from build123d import *

# Parameters (mm, degrees)
F1_W     = 106
F1_H     = 44
F1_W_2   = 100
F1_H_2   = 38
F2_DEPTH = 40
F3_W     = 106
F3_H     = 44
F3_W_2   = 100
F3_H_2   = 38
F4_DEPTH = 3


with BuildPart() as f2:
    # F1 (on Top) → F2 (new body)
    with BuildSketch(Plane.XY):
        Rectangle(F1_W, F1_H)
        Rectangle(F1_W_2, F1_H_2, mode=Mode.SUBTRACT)
    extrude(amount=-F2_DEPTH)

    # F3 (on face) → F4 (join)
    with BuildSketch(Plane(origin=(0, 0, -40), x_dir=(1, 0, 0), z_dir=(0, 0, -1))):
        Rectangle(F3_W, F3_H)
        Rectangle(F3_W_2, F3_H_2, mode=Mode.SUBTRACT)
        Rectangle(F3_W_2, F3_H_2)
    extrude(amount=F4_DEPTH)


solid = f2.part
Can you work these out from the model? Positions are in its coordinate system, mm. A direction names the side the tool comes from. Give positions to 0.01 mm unless a question says otherwise; leave off trailing zeros. Loops run counter-clockwise (first coordinate to the right, second up) from the corner with the lowest first, then second, coordinate; pieces in that order, holes last. Notation, with made-up numbers: (-21, 86) - (14, 86) arc R10 ccw to (14, 99) - close; hole circle Ø1 at (-29.75, -14.75). An arc over 180 degrees is marked (long way). One line per item, written item: value.
(1) If we section it at C-C, the plane x = 23.5: List the corners of the cut face in (y, z) for me.
Verdict:
outline: (-22, -43) - (22, -43) - (22, 0) - (19, 0) - (19, -40) - (-19, -40) - (-19, 0) - (-22, 0) - close
(2) I need wall thicknesses on line 1 along Y through (x, z) = (4, -3); line 2 along X through (y, z) = (-14.5, -6.5); line 3 along Z through (x, y) = (-10, -1.5). Which ranges of each line are inside material? Lowest first, please.
Verdict:
line 1: -22 to -19, 19 to 22
line 2: -53 to -50, 50 to 53
line 3: -43 to -40
(3) If we mould it in two halves opening along X, with no side actions, what happens to faces 3 (the face through (53, 0, -21)), 4 (the face through (-1, 22, -21)), 5 (the face through (-1, 19, -20))? For each: released by +X, released by -X, zero draft, split by the parting line, or undercut.
Verdict:
face 3: released by +X
face 4: zero draft
face 5: undercut
(4) If we section it at B-B, the plane z = -18.5: List the corners of the cut face in (x, y) for me, plus the area to 3 significant figures.
Verdict:
outline: (-53, -22) - (53, -22) - (53, 22) - (-53, 22) - close; hole (-50, -19) - (50, -19) - (50, 19) - (-50, 19) - close
area: 864 mm^2
(5) I'm going to push a flat-ended pin straight in: pin 1 (11.5 mm diameter, centred on x = -21, y = 4, fed in from +Z). Where does the tip first touch, or does it pass through?
Verdict:
pin 1: z = -40
(6) If we section it at A-A, the plane y = 18: List the corners of the cut face in (x, z) for me.
Verdict:
outline: (-53, -43) - (53, -43) - (53, 0) - (50, 0) - (50, -40) - (-50, -40) - (-50, 0) - (-53, 0) - close
(7) On a 3-axis mill with a long thin cutter (end or side, diameter ignored), from which of +Z, -Z, +X, -X, +Y, -Y can I reach the whole of each face in a straight line? I mean faces 1 (the face through (50, 0, -20)), 2 (the face through (-4.2, -19.5, 0)). Say none if no direction works.
Verdict:
face 1: +Z
face 2: +Z, +X, -X, +Y, -Y
